Build history of the part. All positions in model axes, mm. Face numbers are marked on the shaded views. Give positions to 0.01 mm unless a question says otherwise; leave off trailing zeros. Order: outer loops, then holes, each group sorted by start corner. A loop starts at its lowest first (then second) coordinate and runs counter-clockwise, first axis right, second up. Notation, with made-up numbers: (40, -22) -> (54, -22) arc R26 ccw to (54, 10) -> close; hole circle Ø2 at (2, 42). An arc over 180 degrees is marked (long way). Use a Markdown table: item, result. Add a question column.
```python
from build123d import *

# Parameters (mm, degrees)
ESBO_O2_R                = 7.5
RESSALTO_EXTRUS_O1_DEPTH = 8.5
ESBO_O3_R                = 5.75
CORTE_EXTRUS_O1_DEPTH    = 4.5
RESSALTO_EXTRUS_O2_START = -8.5
RESSALTO_EXTRUS_O2_DEPTH = 8.5
RESSALTO_EXTRUS_O3_DEPTH = 3
ESBO_O10_R               = 1.5
CORTE_EXTRUS_O2_DEPTH    = 33.179741965
FILETE2_R                = 3
RESSALTO_EXTRUS_O4_DEPTH = 10
FILETE4_R                = 10
FILETE5_R                = 10


with BuildPart() as part:
    # Esboço2 → Ressalto-extrusão1 (new body)
    with BuildSketch(Plane(origin=(0, 0, 0), x_dir=(1, 0, 0), z_dir=(0, 1, 0))):
        with Locations(Location((0, 0, 0), (0, 0, 270))):
            Circle(ESBO_O2_R)
    extrude(amount=RESSALTO_EXTRUS_O1_DEPTH)

    # Esboço3 → Corte-extrusão1 (cut)
    with BuildSketch(Plane.XZ):
        with Locations(Location((0, 0, 0), (0, 0, 270))):
            Circle(ESBO_O3_R)
    extrude(amount=-CORTE_EXTRUS_O1_DEPTH, mode=Mode.SUBTRACT)

    # Esboço4 → Ressalto-extrusão2 (add)
    with BuildSketch(Plane(origin=(0, 8.5, 0), x_dir=(1, 0, 0), z_dir=(0, 1, 0)).offset(RESSALTO_EXTRUS_O2_START)):
        with BuildLine():
            Line((5, 19), (-5, 19))
            Line((-5, 19), (-5, 5.590169944))
            ThreePointArc((-5, 5.590169944), (0, 7.5), (5, 5.590169944))
            Line((5, 5.590169944), (5, 19))
        make_face()
    extrude(amount=RESSALTO_EXTRUS_O2_DEPTH)

    # Esboço9 → Ressalto-extrusão3 (add)
    with BuildSketch(Plane(origin=(0, 0, -19), x_dir=(-1, 0, 0), z_dir=(0, 0, -1))):
        Polygon((-3.625309941, 7.143055834), (-9.985237601, -13.028057675), (-2.83236047, -15.283351171), (3.527567189, 4.887762338), (-0.053729842, 6), align=None)
    extrude(amount=-RESSALTO_EXTRUS_O3_DEPTH)

    # Esboço10 → Corte-extrusão2 (cut, through all)
    with BuildSketch(Plane(origin=(0, 0, -19), x_dir=(-1, 0, 0), z_dir=(0, 0, -1))):
        with Locations((-5.563236349, -11.800986501)):
            Circle(ESBO_O10_R)
    extrude(amount=-CORTE_EXTRUS_O2_DEPTH, mode=Mode.SUBTRACT)

    # Filete2
    filete2_edges = [part.edges().sort_by_distance(p)[0] for p in [
        (2.83236047, -15.283351171, -17.5),
        (9.985237601, -13.028057675, -17.5),
    ]]
    fillet(filete2_edges, radius=FILETE2_R)

    # Esboço12 → Ressalto-extrusão4 (add)
    with BuildSketch(Plane(origin=(5, 0, 0), x_dir=(0, 0, -1), z_dir=(1, 0, 0))):
        Polygon((16, -1.5), (5.590169944, 0), (16, 0), (19, 0), (19, -1.5), align=None)
    extrude(amount=-RESSALTO_EXTRUS_O4_DEPTH)

    # Filete4
    filete4_edges = [part.edges().sort_by_distance(p)[0] for p in [
        (5, 2.783095989, -17.5),
    ]]
    fillet(filete4_edges, radius=FILETE4_R)

    # Filete5
    # the kernel refuses this fillet: 10 mm, written as the material it adds along each edge
    with BuildSketch(Plane(origin=(-1.513513461, -1.5, -16), x_dir=(-1.0, -1.1428670067616555e-12, 0), z_dir=(0, 0, -1))) as filete5_piece_1_section:
        with BuildLine():
            CenterArc((7.613313945, -9.108748299), FILETE5_R, 114.373472149, 48.126527851)
            Line((-1.923855563, -6.101690304), (-2.114598953, -6.041549144))
            Line((-2.114598953, -6.041549144), (-0.19074339, 0.06014116))
            Line((-0.19074339, 0.06014116), (0, 0.2))
            ThreePointArc((0, 0.2), (1.74324327, 0.2), (3.403949991, 0.182174966))
            Line((3.403949991, 0.182174966), (3.486486539, 0))
        make_face()
    filete5_piece_1 = extrude(amount=3, mode=Mode.PRIVATE)
    filete5_piece_1 = split(filete5_piece_1, bisect_by=Plane(origin=(-1.609257645, -1.741830898, -17.678279033), z_dir=(0, -0.9897772969969367, 0.14262153536348515)), keep=Keep.TOP, mode=Mode.PRIVATE)
    add(filete5_piece_1)
    with BuildSketch(Plane(origin=(-1.513513461, -1.5, -16), x_dir=(-1.0, -1.1428670067616555e-12, 0), z_dir=(0, 0, -1))) as filete5_piece_2_section:
        with BuildLine():
            CenterArc((7.613313945, -9.108748299), FILETE5_R, 114.373472149, 48.126527851)
            Line((-1.923855563, -6.101690304), (-2.114598953, -6.041549144))
            Line((-2.114598953, -6.041549144), (-0.19074339, 0.06014116))
            Line((-0.19074339, 0.06014116), (0, 0.2))
            ThreePointArc((0, 0.2), (1.74324327, 0.2), (3.403949991, 0.182174966))
            Line((3.403949991, 0.182174966), (3.486486539, 0))
        make_face()
    filete5_piece_2 = extrude(amount=3, mode=Mode.PRIVATE)
    filete5_piece_2 = split(filete5_piece_2, bisect_by=Plane(origin=(-3.063320239, -1.747230158, -17.715749287), z_dir=(0, 0.9897772969969367, -0.14262153536348515)), keep=Keep.TOP, mode=Mode.PRIVATE)
    add(filete5_piece_2)
    with BuildSketch(Plane(origin=(-1.513513461, -1.5, -0.00550001), x_dir=(-1.0, -1.1395552717741066e-12, 0), z_dir=(0, 0, -1))) as filete5_piece_3_section:
        with BuildLine():
            CenterArc((7.613313945, -9.108748299), FILETE5_R, 114.373472149, 48.126527851)
            Line((-1.923855563, -6.101690304), (-2.114598953, -6.041549144))
            Line((-2.114598953, -6.041549144), (-0.19074339, 0.06014116))
            Line((-0.19074339, 0.06014116), (0, 0.2))
            ThreePointArc((0, 0.2), (1.74324327, 0.2), (3.403949991, 0.182174966))
            Line((3.403949991, 0.182174966), (3.486486539, 0))
        make_face()
    filete5_piece_3 = extrude(amount=18.99449999, mode=Mode.PRIVATE)
    filete5_piece_3 = split(filete5_piece_3, bisect_by=Plane(origin=(-3.132069725, -1.369378897, -16), z_dir=(0, 0, 1)), keep=Keep.TOP, mode=Mode.PRIVATE)
    filete5_piece_3 = split(filete5_piece_3, bisect_by=Plane(origin=(-3.132069725, -1.433360973, -15.537532703), z_dir=(0, 0.9897772969969367, -0.14262153536348515)), keep=Keep.TOP, mode=Mode.PRIVATE)
    add(filete5_piece_3)


solid = part.part
```
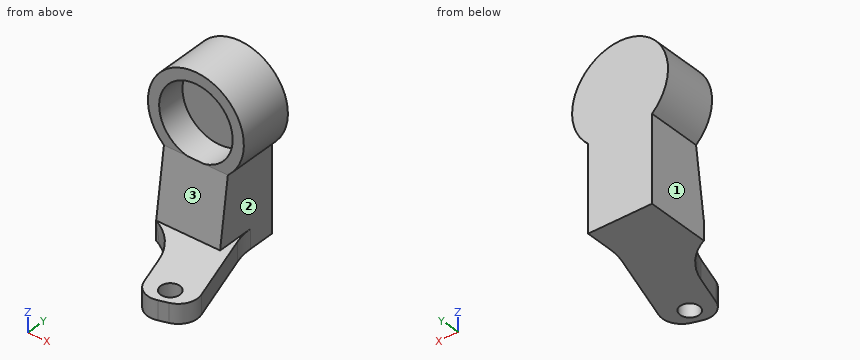
(1) Band-saw the part on A-A on z = 0. Give the cut face in (x, y).
(2) Mould opens along Z. For the marked faces 1, 2 and 3 say: released by +Z, released by -Z, zero draft, split by the parting line, or undercut.
(3) Wall check: probe 1 along X at (y, z) = (2.3, 0); probe 2 along Z at (x, y) = (5.25, 0.75); probe 3 along Y at (x, z) = (5.75, 3.75). Give the ranges that are in metal, low to high.
(4) Band-saw the part on C-C on x = -2.75. Give the cut face in (y, z), plus the area to 3 significant figures.
(5) Pin check, flat tips, straight feed: pin 1 Ø5 at (y, z) = (3, -9) entering from -X; pin 2 Ø4 at (x, z) = (2, -1) entering from -Y; pin 3 Ø6 at (x, y) = (-4.5, 3) entering from +Z; pin 4 Ø4 at (x, y) = (5.5, 3) entering from -Z. Stop position of each tip, or through.
(6) Band-saw the part on D-D on y = 5.25. Give the cut face in (x, z).
(7) Band-saw the part on B-B on y = 2. Give the cut face in (x, z).
Response:
| question | item | result |
|---|---|---|
| 1 | outline | (-7.5, 0) -> (-5.75, 0) -> (-5.75, 4.5) -> (5.75, 4.5) -> (5.75, 0) -> (7.5, 0) -> (7.5, 8.5) -> (-7.5, 8.5) -> close |
| 2 | face 1 | zero draft |
| 2 | face 2 | undercut |
| 2 | face 3 | released by +Z |
| 3 | probe 1 | x = -7.5 to -5.75, 5.75 to 7.5 |
| 3 | probe 2 | z = -19 to -16, -5.36 to -2.35, 2.35 to 5.36 |
| 3 | probe 3 | y = 0 to 8.5 |
| 4 | outline | (-2.91, -19) -> (8.5, -19) -> (8.5, 6.98) -> (0, 6.98) -> (0, 5.05) -> (4.5, 5.05) -> (4.5, -5.05) -> (0, -5.05) -> (0, -5.59) -> (-1.5, -16) -> (-2.91, -16) -> close |
| 4 | area | 192 mm² |
| 5 | pin 1 | stops at x = -5 |
| 5 | pin 2 | stops at y = 4.5 |
| 5 | pin 3 | stops at z = 7.35 |
| 5 | pin 4 | stops at z = -19 |
| 6 | outline | (-5, -19) -> (5, -19) -> (5, -5.59) arc R7.5 ccw (long way) to (-5, -5.59) -> close |
| 7 | outline | (-5, -19) -> (5.27, -19) -> (5.27, -16) -> (5, -16) -> (5, -5.59) arc R7.5 ccw (long way) to (-5, -5.59) -> close; hole circle Ø11.5 at (0, 0) |
